```python
from build123d import *

# Parameters (mm, degrees)
CYLINDER039_R          = 1.5
CYLINDER039_DEPTH      = 1.6
BOX015_W               = 1.8
BOX015_H               = 6
BOX015_DEPTH           = 1
BOX015_PLACEMENT_ANGLE = 5.7
BOX016_W               = 1.8
BOX016_H               = 10
BOX016_DEPTH           = 1
BOX016_PLACEMENT_ANGLE = 5.7
BOX017_W               = 1.8
BOX017_H               = 10
BOX017_DEPTH           = 1
BOX017_PLACEMENT_ANGLE = 5.7
BOX018_W               = 1.8
BOX018_H               = 10
BOX018_DEPTH           = 1
BOX018_PLACEMENT_ANGLE = 5.7
BOX019_W               = 35
BOX019_H               = 30
BOX019_DEPTH           = 1
BOX_W                  = 45
BOX_H                  = 40
BOX_DEPTH              = 1


with BuildPart() as rc522_cyl_col1:
    # Cylinder039 → Cylinder039 (new body)
    with BuildSketch(Plane(origin=(32, -3.4, -6.1), x_dir=(1, 0, 0), z_dir=(0, 0, 1))):
        Circle(CYLINDER039_R)
    extrude(amount=CYLINDER039_DEPTH)


with BuildPart() as rc522_cyl_col004:
    # Clone015 base: copy of rc522-cyl-col1
    add(rc522_cyl_col1.part)


with BuildPart() as rc522_cyl_col004_1:
    # Clone015 placement: moved
    add(rc522_cyl_col004.part.moved(Location((-37.4, 29.7, 0))))


with BuildPart() as rc522_cyl_col003:
    # Clone014 base: copy of rc522-cyl-col1
    add(rc522_cyl_col1.part)


with BuildPart() as rc522_cyl_col003_1:
    # Clone014 placement: moved
    add(rc522_cyl_col003.part.moved(Location((-37.4, 4.7, 0))))


with BuildPart() as rc522_cyl_col002:
    # Clone013 base: copy of rc522-cyl-col1
    add(rc522_cyl_col1.part)


with BuildPart() as rc522_cyl_col002_1:
    # Clone013 placement: moved
    add(rc522_cyl_col002.part.moved(Location((0, 34.4, 0))))


with BuildPart() as cube011:
    # Box015 → Box015 (new body)
    with BuildSketch(Plane.XY):
        with Locations((0.9, 3)):
            Rectangle(BOX015_W, BOX015_H)
    extrude(amount=BOX015_DEPTH)


with BuildPart() as cube011_1:
    # Box015 placement: moved
    add(cube011.part.moved(Location((6.14, 30.65, -7))).rotate(Axis((6.14, 30.65, -7), (0, 0, 1)), BOX015_PLACEMENT_ANGLE))


with BuildPart() as cube012:
    # Box016 → Box016 (new body)
    with BuildSketch(Plane.XY):
        with Locations((0.9, 5)):
            Rectangle(BOX016_W, BOX016_H)
    extrude(amount=BOX016_DEPTH)


with BuildPart() as cube012_1:
    # Box016 placement: moved
    add(cube012.part.moved(Location((29.32, 28.95, -7))).rotate(Axis((29.32, 28.95, -7), (0, 0, 1)), BOX016_PLACEMENT_ANGLE))


with BuildPart() as cube013:
    # Box017 → Box017 (new body)
    with BuildSketch(Plane.XY):
        with Locations((0.9, 5)):
            Rectangle(BOX017_W, BOX017_H)
    extrude(amount=BOX017_DEPTH)


with BuildPart() as cube013_1:
    # Box017 placement: moved
    add(cube013.part.moved(Location((10.55, -13.56, -7))).rotate(Axis((10.55, -13.56, -7), (0, 0, 1)), BOX017_PLACEMENT_ANGLE))


with BuildPart() as cube014:
    # Box018 → Box018 (new body)
    with BuildSketch(Plane.XY):
        with Locations((0.9, 5)):
            Rectangle(BOX018_W, BOX018_H)
    extrude(amount=BOX018_DEPTH)


with BuildPart() as cube014_1:
    # Box018 placement: moved
    add(cube014.part.moved(Location((33.33, -11.25, -7))).rotate(Axis((33.33, -11.25, -7), (0, 0, 1)), BOX018_PLACEMENT_ANGLE))


with BuildPart() as cube015:
    # Box019 → Box019 (new body)
    with BuildSketch(Plane(origin=(-3, -1.16, -7), x_dir=(1, 0, 0), z_dir=(0, 0, 1))):
        with Locations((17.5, 15)):
            Rectangle(BOX019_W, BOX019_H)
    extrude(amount=BOX019_DEPTH)


with BuildPart() as plastic_substrate:
    # Box → Box (new body)
    with BuildSketch(Plane(origin=(-8, -6.16, -7), x_dir=(1, 0, 0), z_dir=(0, 0, 1))):
        with Locations((22.5, 20)):
            Rectangle(BOX_W, BOX_H)
    extrude(amount=BOX_DEPTH)

    # Cut006: cut Cube015
    add(cube015.part, mode=Mode.SUBTRACT)

    # Fusion014: union Cube014
    add(cube014_1.part)

    # Fusion015: union Cube013
    add(cube013_1.part)

    # Fusion016: union Cube012
    add(cube012_1.part)

    # Fusion017: union Cube011
    add(cube011_1.part)

    # Fusion018: union rc522-cyl-col1
    add(rc522_cyl_col1.part)

    # Fusion019: union rc522-cyl-col002
    add(rc522_cyl_col002_1.part)

    # Fusion020: union rc522-cyl-col003
    add(rc522_cyl_col003_1.part)

    # Fusion021: union rc522-cyl-col004
    add(rc522_cyl_col004_1.part)


with BuildPart() as plastic_substrate_1:
    # Fusion021 placement: moved
    add(plastic_substrate.part.moved(Location((-2.54, 0, 0))))


solid = plastic_substrate_1.part
```
Geometry check sheet. Reference: the model listing, model coordinates, mm. A direction names the side the tool comes from. Give positions to 0.01 mm unless a question says otherwise; leave off trailing zeros. Order: outer loops, then holes, each group sorted by start corner. A loop starts at its lowest first (then second) coordinate and runs counter-clockwise, first axis right, second up. Notation, with made-up numbers: (31.25, 1) - (50.25, 1) arc R14 ccw to (50.25, 27) - close; hole circle Ø9 at (50, 20). An arc over 180 degrees is marked (long way). Write item = value, one per line. Start each with the question number.
1) Scan lines: L1, parallel to Y at x = 19, z = -6.3; L2, parallel to X at y = 24, z = -6.1; L3, parallel to Y at x = 29.5, z = -6.9. Record each from-to range of solid material in increasing order.
2) Access from +Z, -Z, +X, -X, +Y, -Y to the whole of each face (thin tool, end or side, straight path). Record for faces 4 (the flat face through (29, 31, -4.5)), 5 (the cylindrical face through (-9.44, 26.37, -5.26)).
3) Gauge pin test, flat ends, axial feed: pin 1 Ø0.8 at (x, z) = (15, -6.5) entering from -Y; pin 2 Ø0.5 at (x, z) = (-3.5, -6.5) entering from +Y; pin 3 Ø6 at (x, y) = (25.5, 14.5) entering from +Z; pin 4 Ø13.5 at (x, y) = (14, 24) entering from +Z. Record the tip position at first contact, or that the pin passes through.
4) Section check C-C (x = 13.5). Enter the section's corners in (y, z).
5) Section check A-A (y = 1.3). Enter the section's corners in (x, z), then the cut area to 3 significant figures.
6) Draft check along Y on faces 1 (the cylindrical face through (27.96, 31.07, -5.26)), 2 (the flat face through (13, -3, -7)), 3 (the cylindrical face through (27.96, -3.33, -5.26)). Enter one of: released by +Y, released by -Y, zero draft, split by the parting line, or undercut.
7) Section check B-B (z = -6.5). Enter the section's corners in (x, y).
8) Section check D-D (y = 7.5). Enter the section's corners in (x, z), then the cut area to 3 significant figures.
Geometry check:
q1.L1 = -6.16 to -1.16, 28.84 to 33.84
q1.L2 = -10.54 to -5.54, 29.46 to 34.46
q1.L3 = -6.16 to 33.84
q2.face_4 = +Z, +X, -X, +Y, -Y
q2.face_5 = +Z
q3.pin_1 = -6.16
q3.pin_2 = 33.84
q3.pin_3 = through
q3.pin_4 = -6
q4.outline = (-6.16, -7) - (-1.16, -7) - (-1.16, -6) - (-6.16, -6) - close; (28.84, -7) - (33.84, -7) - (33.84, -6) - (28.84, -6) - close
q5.outline = (-10.54, -7) - (-5.54, -7) - (-5.54, -6) - (-6.44, -6) - (-6.44, -4.5) - (-9.44, -4.5) - (-9.44, -6) - (-10.54, -6) - close; (29.46, -7) - (34.46, -7) - (34.46, -6) - (29.46, -6) - close
q5.area = 14.5 mm2
q6.face_1 = undercut
q6.face_2 = zero draft
q6.face_3 = undercut
q7.outline = (-10.54, -6.16) - (7.27, -6.16) - (8.01, -13.56) - (9.8, -13.38) - (9.08, -6.16) - (30.28, -6.16) - (30.79, -11.25) - (32.58, -11.07) - (32.09, -6.16) - (34.46, -6.16) - (34.46, 33.84) - (28.1, 33.84) - (27.58, 39.08) - (25.79, 38.9) - (26.29, 33.84) - (5.09, 33.84) - (4.8, 36.8) - (3, 36.62) - (3.28, 33.84) - (-10.54, 33.84) - close; hole (-5.54, -1.16) - (29.46, -1.16) - (29.46, 28.84) - (-5.54, 28.84) - close
q8.outline = (-10.54, -7) - (-5.54, -7) - (-5.54, -6) - (-10.54, -6) - close; (29.46, -7) - (34.46, -7) - (34.46, -6) - (29.46, -6) - close
q8.area = 10.0 mm2
